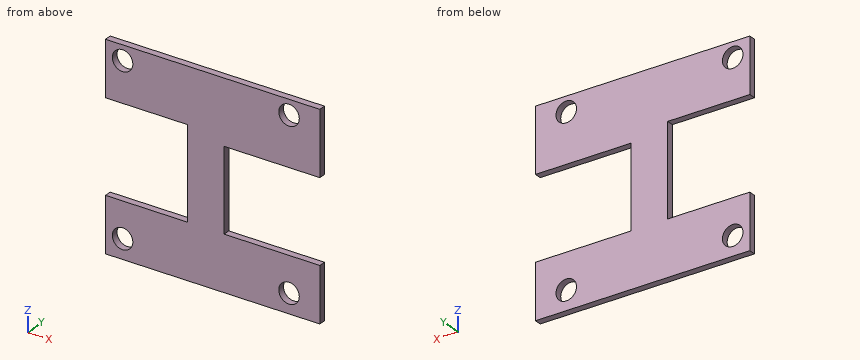
from build123d import *

# Parameters (mm, degrees)
BOX002_W               = 21
BOX002_H               = 18
BOX002_DEPTH           = 10
BOX001_W               = 18
BOX001_H               = 20
BOX001_DEPTH           = 10
CYLINDER002_R          = 2.25
CYLINDER002_DEPTH      = 10
CYLINDER003_R          = 2.25
CYLINDER003_DEPTH      = 10
CYLINDER004_R          = 2.25
CYLINDER004_DEPTH      = 10
CYLINDER005_R          = 2.25
CYLINDER005_DEPTH      = 10
BOX_W                  = 44
BOX_H                  = 47
BOX_DEPTH              = 1.5
CUT001_PLACEMENT_ANGLE = 90


with BuildPart() as obj1:
    # Box002 → Box002 (new body)
    with BuildSketch(Plane(origin=(-21, 12, -1), x_dir=(1, 0, 0), z_dir=(0, 0, 1))):
        with Locations((10.5, 9)):
            Rectangle(BOX002_W, BOX002_H)
    extrude(amount=BOX002_DEPTH)


with BuildPart() as compound001:
    # Box001 → Box001 (new body)
    with BuildSketch(Plane(origin=(-47, 12, -1), x_dir=(1, 0, 0), z_dir=(0, 0, 1))):
        with Locations((9, 10)):
            Rectangle(BOX001_W, BOX001_H)
    extrude(amount=BOX001_DEPTH)

    # Compound001: union obj1
    add(obj1.part)


with BuildPart() as zylinder002:
    # Cylinder002 → Cylinder002 (new body)
    with BuildSketch(Plane(origin=(-6.75, 4.25, -1), x_dir=(1, 0, 0), z_dir=(0, 0, 1))):
        Circle(CYLINDER002_R)
    extrude(amount=CYLINDER002_DEPTH)


with BuildPart() as zylinder003:
    # Cylinder003 → Cylinder003 (new body)
    with BuildSketch(Plane(origin=(-43.25, 4.25, -1), x_dir=(1, 0, 0), z_dir=(0, 0, 1))):
        Circle(CYLINDER003_R)
    extrude(amount=CYLINDER003_DEPTH)


with BuildPart() as zylinder004:
    # Cylinder004 → Cylinder004 (new body)
    with BuildSketch(Plane(origin=(-6.75, 40.75, -1), x_dir=(1, 0, 0), z_dir=(0, 0, 1))):
        Circle(CYLINDER004_R)
    extrude(amount=CYLINDER004_DEPTH)


with BuildPart() as compound:
    # Cylinder005 → Cylinder005 (new body)
    with BuildSketch(Plane(origin=(-43.25, 40.75, -1), x_dir=(1, 0, 0), z_dir=(0, 0, 1))):
        Circle(CYLINDER005_R)
    extrude(amount=CYLINDER005_DEPTH)

    # Compound: union Zylinder002, Zylinder003, Zylinder004
    add(zylinder002.part)
    add(zylinder003.part)
    add(zylinder004.part)


with BuildPart() as cut001:
    # Box → Box (new body)
    with BuildSketch(Plane(origin=(0, 0, 0), x_dir=(0, 1, 0), z_dir=(0, 0, 1))):
        with Locations((22, 23.5)):
            Rectangle(BOX_W, BOX_H)
    extrude(amount=BOX_DEPTH)

    # Cut: cut Compound
    add(compound.part, mode=Mode.SUBTRACT)

    # Cut001: cut Compound001
    add(compound001.part, mode=Mode.SUBTRACT)


with BuildPart() as cut001_1:
    # Cut001 placement: moved
    add(cut001.part.moved(Location((23.5, 2, 9))).rotate(Axis((23.5, 2, 9), (1, 0, 0)), CUT001_PLACEMENT_ANGLE))


solid = cut001_1.part
Work out the finished part from the listing and answer in its coordinate system (mm). Coordinates: 2 decimals unless noted, no trailing zeros. Write each loop counter-clockwise with the first axis right and the second up, starting at its lowest first coordinate (ties: lowest second). Pieces come first, ordered by that corner, then holes. Notation, with made-up numbers: M 66,-28.75 L 124,-28.75 A19 ccw 124,-5.75 Z; hole C 2.5,89 d3. An arc over 180 degrees is marked long. Answer as CSV lines item,"result". Start each with the question number.
Item 1: Section C-C on y = 1.45 is taken. Write down the section's boundary in (x, z), and give its area (3 significant figures).
Item 2: Section B-B on z = 13.25 is taken. Write down the section's boundary in (x, y), and give its area (3 significant figures).
Item 3: Section D-D on x = -19.75 is taken. Write down the section's boundary in (y, z), and give its area (3 significant figures).
Item 4: Flat-ended cylindrical pins translate along their axes: P1, Ø2.5, axis at x = -19.75, z = 13.25, coming from the -Y side; P2, Ø0.8, axis at y = 1.5, z = 26.5, coming from the +X side. Find the tip coordinate at first contact, or state that the pin passes through.
Item 5: Consider L1, parallel to Z at x = 16.75, y = 1.75; L2, parallel to X at y = 1.3, z = 49.75; L3, parallel to Z at x = 10, y = 1.15. Determine where each line is inside the solid, lowest interval first.
Item 6: Section A-A on x = -7.5 is taken. Write down the section's boundary in (y, z).
Checks:
1,outline,"M -23.5,9 L 23.5,9 L 23.5,21 L 2.5,21 L 2.5,39 L 23.5,39 L 23.5,53 L -23.5,53 L -23.5,41 L -5.5,41 L -5.5,21 L -23.5,21 Z; hole C -19.75,13.25 d4.5; hole C -19.75,49.75 d4.5; hole C 16.75,13.25 d4.5; hole C 16.75,49.75 d4.5"
1,area,"1,270 mm²"
2,outline,"M -23.5,0.5 L -22,0.5 L -22,2 L -23.5,2 Z; M -17.5,0.5 L 14.5,0.5 L 14.5,2 L -17.5,2 Z; M 19,0.5 L 23.5,0.5 L 23.5,2 L 19,2 Z"
2,area,"57.0 mm²"
3,outline,"M 0.5,9 L 2,9 L 2,11 L 0.5,11 Z; M 0.5,15.5 L 2,15.5 L 2,21 L 0.5,21 Z; M 0.5,41 L 2,41 L 2,47.5 L 0.5,47.5 Z; M 0.5,52 L 2,52 L 2,53 L 0.5,53 Z"
3,area,"22.5 mm²"
4,P1,"passes through"
4,P2,"stops at x = 2.5"
5,L1,"z = 9 to 11, 15.5 to 21, 39 to 47.5, 52 to 53"
5,L2,"x = -23.5 to -22, -17.5 to 14.5, 19 to 23.5"
5,L3,"z = 9 to 21, 39 to 53"
6,outline,"M 0.5,9 L 2,9 L 2,21 L 0.5,21 Z; M 0.5,41 L 2,41 L 2,53 L 0.5,53 Z"
